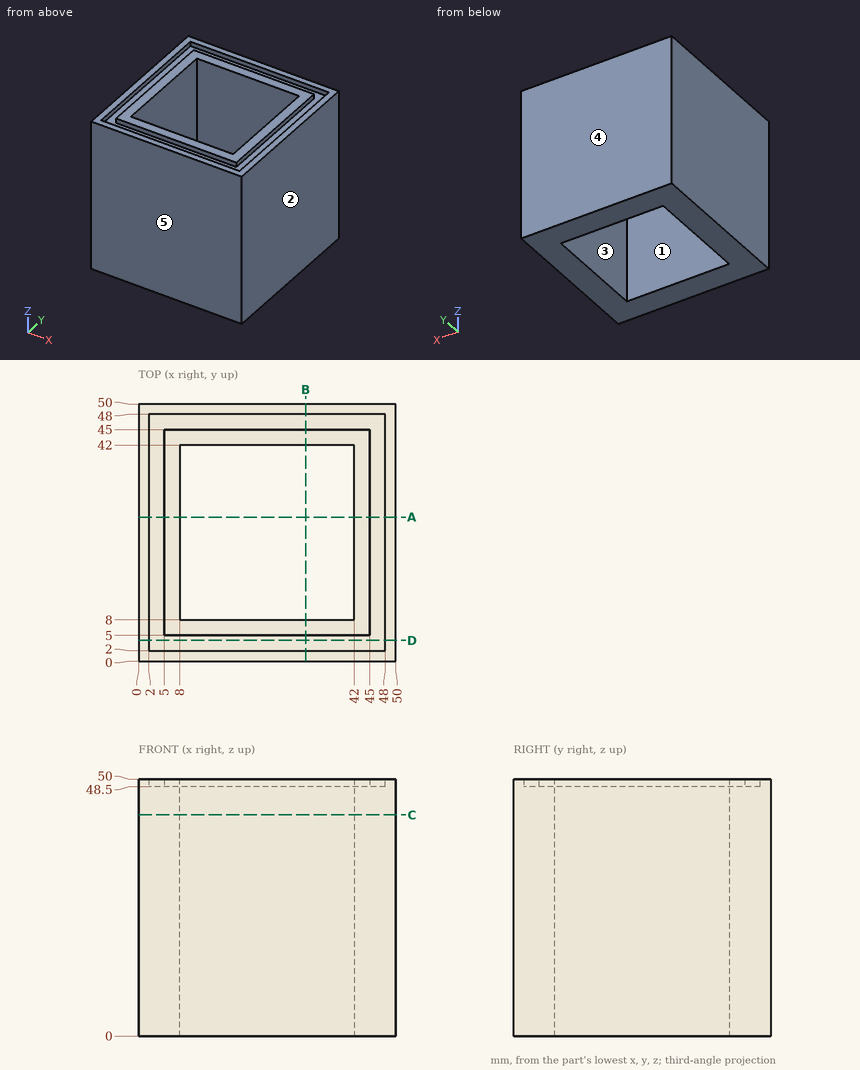
Drawing for the job (mm, zero at the part's lowest x, y, z). A direction names the side the tool comes from. Give positions to 0.01 mm unless a question says otherwise; leave off trailing zeros. Order: outer loops, then holes, each group sorted by start corner. A loop starts at its lowest first (then second) coordinate and runs counter-clockwise, first axis right, second up. Notation, with made-up numbers: M -32.75,32 L 11.25,32 A7 cw 11.25,41 Z; hole C 18,39.5 d8. An arc over 180 degrees is marked long. Write item = value, one per line. Start each with the question number.
(1) Slice it at A-A on y = 28. Write the cut outline in (x, z).
(2) Slice it at D-D on y = 4. Write the cut outline in (x, z), plus the area to 3 significant figures.
(3) Probe L1, parallel to X at y = 15, z = 42.5; L2, parallel to Z at x = 47.5, y = 22.5. List the from-to ranges inside material, lowest first. Write a range as [from, to].
(4) Which spindle directions (+Z, -Z, +X, -X, +Y, -Y) get a long thin tool onto all of the face, cutting with end or side? Do the marked faces 1 and 2. Say none if no direction does.
(5) Two-plate mould, pull along Y, no slides. Class the marked faces 3, 4 and 5: released by +Y, released by -Y, zero draft, split by the parting line, or undercut.
(6) Slice it at C-C on z = 43. Write the cut outline in (x, y), plus the area to 3 significant figures.
Responses:
q1.outline = M 0,0 L 8,0 L 8,50 L 5,50 L 5,48.5 L 2,48.5 L 2,50 L 0,50 Z; M 42,0 L 50,0 L 50,50 L 48,50 L 48,48.5 L 45,48.5 L 45,50 L 42,50 Z
q2.outline = M 0,0 L 50,0 L 50,50 L 48,50 L 48,48.5 L 2,48.5 L 2,50 L 0,50 Z
q2.area = 2,430 mm2
q3.L1 = [0, 8], [42, 50]
q3.L2 = [0, 48.5]
q4.face_1 = +Z, -Z
q4.face_2 = +Z, -Z, +X, +Y, -Y
q5.face_3 = undercut
q5.face_4 = released by +Y
q5.face_5 = released by -Y
q6.outline = M 0,0 L 50,0 L 50,50 L 0,50 Z; hole M 8,8 L 42,8 L 42,42 L 8,42 Z
q6.area = 1,340 mm2
